Build history of the part. All positions in model axes, mm. A direction names the side the tool comes from. Round coordinates to 2 decimals unless told otherwise and drop trailing zeros. Order: outer loops, then holes, each group sorted by start corner. A loop starts at its lowest first (then second) coordinate and runs counter-clockwise, first axis right, second up. Notation, with made-up numbers: (79.25, 4) -> (117.25, 4) arc R26 ccw to (117.25, 23) -> close; hole circle Ø6 at (65, 70). An arc over 180 degrees is marked (long way). Write item = value, one per line.
from build123d import *

# Parameters (mm, degrees)
SKETCH051_R                = 2.875
SKETCH051_R_2              = 1.625
EXTRUDE049_DEPTH           = 13
EXTRUDE049_PLACEMENT_ANGLE = 270
SKETCH050_R                = 1.625
EXTRUDE048_DEPTH           = 4
EXTRUDE048_PLACEMENT_ANGLE = 270
FILLET040_R                = 1


with BuildPart() as spacer001:
    # Sketch051 → Extrude049 (new body)
    with BuildSketch(Plane.YZ):
        with Locations((3, 38.75)):
            Circle(SKETCH051_R)
        with Locations((3, 38.75)):
            Circle(SKETCH051_R_2, mode=Mode.SUBTRACT)
        with Locations((3, 3)):
            Circle(SKETCH051_R)
        with Locations((3, 3)):
            Circle(SKETCH051_R_2, mode=Mode.SUBTRACT)
        with Locations((103.75, 3)):
            Circle(SKETCH051_R)
        with Locations((103.75, 3)):
            Circle(SKETCH051_R_2, mode=Mode.SUBTRACT)
        with Locations((103.75, 38.75)):
            Circle(SKETCH051_R)
        with Locations((103.75, 38.75)):
            Circle(SKETCH051_R_2, mode=Mode.SUBTRACT)
    extrude(amount=EXTRUDE049_DEPTH)


with BuildPart() as spacer001_1:
    # Extrude049 placement: moved
    add(spacer001.part.moved(Location((0, -2, 0))).rotate(Axis((0, -2, 0), (0, 0, 1)), EXTRUDE049_PLACEMENT_ANGLE))


with BuildPart() as top_fillet001:
    # Sketch050 → Extrude048 (new body)
    with BuildSketch(Plane.YZ):
        Polygon((106.25, 0), (106.25, 41.75), (0, 41.75), (0, 0), (18.25, 0), (18.25, 15), (88, 15), (88, 0), align=None)
        with Locations((3, 3)):
            Circle(SKETCH050_R, mode=Mode.SUBTRACT)
        with Locations((3, 38.75)):
            Circle(SKETCH050_R, mode=Mode.SUBTRACT)
        with Locations((103.75, 38.75)):
            Circle(SKETCH050_R, mode=Mode.SUBTRACT)
        with Locations((103.75, 3)):
            Circle(SKETCH050_R, mode=Mode.SUBTRACT)
    extrude(amount=EXTRUDE048_DEPTH)


with BuildPart() as top_fillet001_1:
    # Extrude048 placement: moved
    add(top_fillet001.part.moved(Location((0, -15, 0))).rotate(Axis((0, -15, 0), (0, 0, 1)), EXTRUDE048_PLACEMENT_ANGLE))

    # Fusion077: union spacer001
    add(spacer001_1.part)

    # Fillet040
    fillet040_edges = [top_fillet001_1.edges().sort_by_distance(p)[0] for p in [
        (106.25, -17, 0),
        (106.25, -17, 41.75),
        (88, -17, 0),
        (0, -17, 41.75),
        (88, -17, 15),
        (0, -17, 0),
        (18.25, -17, 15),
        (18.25, -17, 0),
    ]]
    fillet(fillet040_edges, radius=FILLET040_R)


solid = top_fillet001_1.part
Q1. Flat gauge pins, fed straight in: pin 1 (4 mm diameter, centred on x = 11, y = -12.5, fed in from -Z); pin 2 (3 mm diameter, centred on y = -16.5, z = 6.5, fed in from +X); pin 3 (3 mm diameter, centred on x = 46.5, y = -16.5, fed in from -Z); pin 4 (6 mm diameter, centred on y = -4.5, z = 6, fed in from -X) (3 decimals). Where does each tip first touch, or does it go through?
Check values:
pin_1 = through
pin_2 = 106.25
pin_3 = 15
pin_4 = 0.125
Q2. Cut at B-B, the plane z = 3. List the corners of the cut face in (x, y) (3 decimals), and give its area (3 significant figures).
Check values:
outline = (0, -19) -> (1.375, -19) -> (1.375, -2) -> (0.125, -2) -> (0.125, -15) -> (0, -15) -> close; (4.625, -19) -> (18.25, -19) -> (18.25, -15) -> (5.875, -15) -> (5.875, -2) -> (4.625, -2) -> close; (88, -19) -> (102.125, -19) -> (102.125, -2) -> (100.875, -2) -> (100.875, -15) -> (88, -15) -> close; (105.375, -19) -> (106.25, -19) -> (106.25, -15) -> (106.625, -15) -> (106.625, -2) -> (105.375, -2) -> close
area = 185 mm²
Q3. Cut at D-D, the plane x = 103.75. List the corners of the cut face in (y, z) (3 decimals).
Check values:
outline = (-19, 0) -> (-15, 0) -> (-15, 0.125) -> (-2, 0.125) -> (-2, 1.375) -> (-19, 1.375) -> close; (-19, 4.625) -> (-2, 4.625) -> (-2, 5.875) -> (-15, 5.875) -> (-15, 35.875) -> (-2, 35.875) -> (-2, 37.125) -> (-19, 37.125) -> close; (-19, 40.375) -> (-2, 40.375) -> (-2, 41.625) -> (-15, 41.625) -> (-15, 41.75) -> (-19, 41.75) -> close
Q4. Which spindle directions (+Z, -Z, +X, -X, +Y, -Y) get a long thin tool onto all of the face, cutting with end or side? Do faces 4 (the face through (3.874, -10.381, 4.37)), 5 (the face through (53, -17, 15)), 6 (the face through (106.492, -8.409, 3.864)), 7 (the face through (106.25, -17, 21)). Say none if no direction does.
Check values:
face_4 = +Y, -Y
face_5 = -Z, +Y, -Y
face_6 = +Y
face_7 = +Z, -Z, +X, -Y
Q5. Probe probe 1 along Z at (x, y) = (3, -13) (3 decimals); probe 2 along Y at (x, z) = (12, 12); probe 3 along X at (y, z) = (-7.75, 5.5). List the from-to ranges inside material, lowest first.
Check values:
probe_1 = 0.125 to 1.375, 4.625 to 5.875, 35.875 to 37.125, 40.375 to 41.625
probe_2 = -19 to -15
probe_3 = 1.58 to 4.42, 102.33 to 105.17
Q6. Cut at A-A, the plane y = -5.25. List the corners of the cut face in (x, z) (3 decimals).
Check values:
outline = circle Ø5.75 at (3, 3); circle Ø5.75 at (3, 38.75); circle Ø5.75 at (103.75, 3); circle Ø5.75 at (103.75, 38.75); hole circle Ø3.25 at (3, 3); hole circle Ø3.25 at (3, 38.75); hole circle Ø3.25 at (103.75, 3); hole circle Ø3.25 at (103.75, 38.75)
Q7. Mould opens along X. For faces 1 (the face through (18.25, -17, 7)), 2 (the face through (103.7, -2, 36.9)), 3 (the face through (0, -17, 21)) say: released by +X, released by -X, zero draft, split by the parting line, or undercut.
Check values:
face_1 = undercut
face_2 = zero draft
face_3 = released by -X
Q8. Cut at C-C, the plane y = -17. List the corners of the cut face in (x, z) (3 decimals), and give its area (3 significant figures).
Check values:
outline = (0, 1) arc R1 ccw to (1, 0) -> (17.25, 0) arc R1 ccw to (18.25, 1) -> (18.25, 14) arc R1 cw to (19.25, 15) -> (87, 15) arc R1 cw to (88, 14) -> (88, 1) arc R1 ccw to (89, 0) -> (105.25, 0) arc R1 ccw to (106.25, 1) -> (106.25, 40.75) arc R1 ccw to (105.25, 41.75) -> (1, 41.75) arc R1 ccw to (0, 40.75) -> close; hole circle Ø3.25 at (3, 3); hole circle Ø3.25 at (3, 38.75); hole circle Ø3.25 at (103.75, 3); hole circle Ø3.25 at (103.75, 38.75)
area = 3,360 mm²
